```python
from build123d import *

# Parameters (mm, degrees)
SKETCH1_W                = 2
SKETCH1_H                = 27
M4_CLEARANCE_HOLE1_D     = 4.5
M4_CLEARANCE_HOLE1_DEPTH = 4.5
CUT_EXTRUDE1_START       = -10
CUT_EXTRUDE1_DEPTH       = 4
CIRPATTERN3_COUNT        = 6
SKETCH7_W                = 13.590111476
SKETCH7_H                = 85.87559673
CUT_EXTRUDE2_DEPTH       = 5
FILLET1_R                = 5
CUT_EXTRUDE3_DEPTH       = 46
BOSS_EXTRUDE1_START      = -9.8884
SKETCH8_3_R              = 2.45
BOSS_EXTRUDE1_DEPTH      = 1
BOSS_EXTRUDE2_START      = -8.8884
SKETCH8_4_R              = 2.45
BOSS_EXTRUDE2_DEPTH      = 4
BOSS_EXTRUDE3_DEPTH      = 37
BOSS_EXTRUDE4_START      = -2
SKETCH12_R               = 2.25
BOSS_EXTRUDE4_DEPTH      = 10


with BuildPart() as part:
    # Sketch1 → Revolve1 (revolve)
    with BuildSketch(Plane.XY):
        Polygon((32.5, 0), (39.5, 0), (52, 0), (52, 4.5), (39.5, 4.5), (39.5, 35), (42.5, 35), (42.5, 45), (32.5, 45), (32.5, 38), (32.5, 33), (32.5, 27), align=None)
        with Locations((31.5, 13.5)):
            Rectangle(SKETCH1_W, SKETCH1_H)
    revolve(axis=Axis((0, 0, 0), (0, 1, 0)))

    # M4 Clearance Hole1
    with Locations(Plane(origin=(0, 4.5, 0), x_dir=(1, 0, 0), z_dir=(0, 1, 0))):
        with Locations((45.75, 0)):
            m4_clearance_hole1 = Hole(M4_CLEARANCE_HOLE1_D / 2, depth=M4_CLEARANCE_HOLE1_DEPTH)

    # Sketch5 → M3 Clearance Hole1 (revolve, cut)
    with BuildSketch(Plane(origin=(35.7, 45, 0), x_dir=(0, 0, 1), z_dir=(1, 0, 0))):
        Polygon((0, 0), (0, 11.021463052), (1.7, 10), (1.7, 0), align=None)
    m3_clearance_hole1 = revolve(axis=Axis((35.7, 51.35, 0), (0, -1, 0)), mode=Mode.SUBTRACT)

    # Sketch4_2 → Cut-Extrude1 (cut)
    with BuildSketch(Plane(origin=(0, 45, 0), x_dir=(1, 0, 0), z_dir=(0, 1, 0)).offset(CUT_EXTRUDE1_START)):
        with BuildLine():
            Line((38.45, 1.58771324), (38.45, -1.58771324))
            Line((38.45, -1.58771324), (35.7, -3.175426481))
            Line((35.7, -3.175426481), (42.214154639, -4.920888955))
            ThreePointArc((42.214154639, -4.920888955), (42.428478479, -2.464592039), (42.5, 0))
            ThreePointArc((42.5, 0), (42.428478479, 2.464592039), (42.214154639, 4.920888955))
            Line((42.214154639, 4.920888955), (35.7, 3.175426481))
            Line((35.7, 3.175426481), (38.45, 1.58771324))
        make_face()
        Polygon((32.95, -1.58771324), (35.7, -3.175426481), (38.45, -1.58771324), (38.45, 1.58771324), (35.7, 3.175426481), (32.95, 1.58771324), align=None)
    cut_extrude1 = extrude(amount=-CUT_EXTRUDE1_DEPTH, mode=Mode.SUBTRACT)

    # CirPattern3: M4 Clearance Hole1, M3 Clearance Hole1, Cut-Extrude1 ×6 about axis
    cirpattern3_axis = Axis((0, 0, 0), (0, 1, 0))
    for i in range(1, CIRPATTERN3_COUNT):
        add(m4_clearance_hole1.rotate(cirpattern3_axis, i * 360 / CIRPATTERN3_COUNT), mode=Mode.SUBTRACT)
        add(m3_clearance_hole1.rotate(cirpattern3_axis, i * 360 / CIRPATTERN3_COUNT), mode=Mode.SUBTRACT)
        add(cut_extrude1.rotate(cirpattern3_axis, i * 360 / CIRPATTERN3_COUNT), mode=Mode.SUBTRACT)

    # Sketch7 → Cut-Extrude2 (cut)
    with BuildSketch(Plane.XZ):
        with Locations((0, -42.937798365)):
            Rectangle(SKETCH7_W, SKETCH7_H)
    extrude(amount=-CUT_EXTRUDE2_DEPTH, mode=Mode.SUBTRACT)

    # Fillet1
    fillet1_edges = [part.edges().sort_by_distance(p)[0] for p in [
        (-6.795055738, 2.5, -29.733436019),
        (-6.795055738, 2.25, -51.554119307),
        (6.795055738, 2.5, -29.733436019),
        (6.795055738, 2.25, -51.554119307),
    ]]
    fillet(fillet1_edges, radius=FILLET1_R)

    # Sketch8 → Cut-Extrude3 (cut, through all)
    with BuildSketch(Plane(origin=(0, 45, 0), x_dir=(1, 0, 0), z_dir=(0, 1, 0))):
        Polygon((-33.77753348, 6.841230885), (-24.786528121, 58.870086558), (-44.494427997, 62.275770406), (-53.485433356, 10.246914732), align=None)
    extrude(amount=-CUT_EXTRUDE3_DEPTH, mode=Mode.SUBTRACT)

    # Sketch8_3 → Boss-Extrude1 (add)
    with BuildSketch(Plane(origin=(0, 45, 0), x_dir=(1, 0, 0), z_dir=(0, 1, 0)).offset(BOSS_EXTRUDE1_START)):
        Polygon((-34.67678822, 54.490274326), (-25.808233276, 52.957716595), (-24.786528121, 58.870086558), (-33.655083065, 60.402644289), align=None)
        with Locations((-30.040674072, 57.240991616)):
            Circle(SKETCH8_3_R, mode=Mode.SUBTRACT)
        Polygon((-45.516133152, 56.363400443), (-36.647578207, 54.830842711), (-35.625873053, 60.743212674), (-44.494427997, 62.275770406), align=None)
        with Locations((-40.091703009, 58.977890378)):
            Circle(SKETCH8_3_R, mode=Mode.SUBTRACT)
        Polygon((-53.485433356, 10.246914732), (-44.616878412, 8.714357001), (-43.595173257, 14.626726964), (-52.463728201, 16.159284695), align=None)
        with Locations((-48.231287405, 11.876009674)):
            Circle(SKETCH8_3_R, mode=Mode.SUBTRACT)
        with BuildLine():
            Line((-41.699432083, 8.210198775), (-33.77753348, 6.841230885))
            Line((-33.77753348, 6.841230885), (-32.755828325, 12.753600847))
            Line((-32.755828325, 12.753600847), (-40.118843779, 14.025989228))
            ThreePointArc((-40.118843779, 14.025989228), (-41.01235693, 11.146146378), (-41.699432083, 8.210198775))
        make_face()
        with Locations((-38.180258468, 10.139110912)):
            Circle(SKETCH8_3_R, mode=Mode.SUBTRACT)
    extrude(amount=BOSS_EXTRUDE1_DEPTH)

    # Sketch8_4 → Boss-Extrude2 (add)
    with BuildSketch(Plane(origin=(0, 45, 0), x_dir=(1, 0, 0), z_dir=(0, 1, 0)).offset(BOSS_EXTRUDE2_START)):
        Polygon((-34.67678822, 54.490274326), (-25.808233276, 52.957716595), (-24.786528121, 58.870086558), (-33.655083065, 60.402644289), align=None)
        with Locations((-30.040674072, 57.240991616)):
            Circle(SKETCH8_4_R, mode=Mode.SUBTRACT)
        Polygon((-45.516133152, 56.363400443), (-36.647578207, 54.830842711), (-35.625873053, 60.743212674), (-44.494427997, 62.275770406), align=None)
        with Locations((-40.091703009, 58.977890378)):
            Circle(SKETCH8_4_R, mode=Mode.SUBTRACT)
        Polygon((-36.647578207, 54.830842711), (-34.67678822, 54.490274326), (-33.655083065, 60.402644289), (-35.625873053, 60.743212674), align=None)
        Polygon((-53.485433356, 10.246914732), (-44.616878412, 8.714357001), (-43.595173257, 14.626726964), (-52.463728201, 16.159284695), align=None)
        with Locations((-48.231287405, 11.876009674)):
            Circle(SKETCH8_4_R, mode=Mode.SUBTRACT)
        Polygon((-44.616878412, 8.714357001), (-42.646088424, 8.373788616), (-41.62438327, 14.286158579), (-43.595173257, 14.626726964), align=None)
        with BuildLine():
            Line((-41.699432083, 8.210198775), (-33.77753348, 6.841230885))
            Line((-33.77753348, 6.841230885), (-32.755828325, 12.753600847))
            Line((-32.755828325, 12.753600847), (-40.118843779, 14.025989228))
            ThreePointArc((-40.118843779, 14.025989228), (-41.01235693, 11.146146378), (-41.699432083, 8.210198775))
        make_face()
        with Locations((-38.180258468, 10.139110912)):
            Circle(SKETCH8_4_R, mode=Mode.SUBTRACT)
        with BuildLine():
            Line((-42.646088424, 8.373788616), (-41.699432083, 8.210198775))
            ThreePointArc((-41.699432083, 8.210198775), (-41.01235693, 11.146146378), (-40.118843779, 14.025989228))
            Line((-40.118843779, 14.025989228), (-41.62438327, 14.286158579))
            Line((-41.62438327, 14.286158579), (-42.646088424, 8.373788616))
        make_face()
    extrude(amount=BOSS_EXTRUDE2_DEPTH)

    # Sketch11 → Boss-Extrude3 (add)
    with BuildSketch(Plane.XZ):
        with BuildLine():
            Line((-27.313133013, -44.249212027), (-24.786528121, -58.870086558))
            Line((-24.786528121, -58.870086558), (-9.274181519, -49.813905189))
            ThreePointArc((-9.274181519, -49.813905189), (-11.110324868, -50.448789631), (-13.049848902, -50.335886241))
            ThreePointArc((-13.049848902, -50.335886241), (-20.409666288, -47.827246649), (-27.313133013, -44.249212027))
        make_face()
    extrude(amount=-BOSS_EXTRUDE3_DEPTH)

    # Sketch12 → Boss-Extrude4 (add)
    with BuildSketch(Plane(origin=(0, 37, 0), x_dir=(1, 0, 0), z_dir=(0, 1, 0)).offset(BOSS_EXTRUDE4_START)):
        with BuildLine():
            ThreePointArc((-6.795055738, 45.495897179), (-7.45890719, 47.985438456), (-9.274182045, 49.813905496))
            Line((-9.274182045, 49.813905496), (-24.786528121, 58.870086558))
            Line((-24.786528121, 58.870086558), (-30.655076171, 24.910164692))
            ThreePointArc((-30.655076171, 24.910164692), (-19.990871879, 34.067800655), (-6.795055738, 38.911145158))
            Line((-6.795055738, 38.911145158), (-6.795055738, 45.495897179))
        make_face()
        with Locations((-22.875, 39.620662223)):
            Circle(SKETCH12_R, mode=Mode.SUBTRACT)
    extrude(amount=BOSS_EXTRUDE4_DEPTH)


solid = part.part
```
Source: CAD feature listing. Evaluate the final solid. Frame: model axes, mm. A direction names the side the tool comes from. Round coordinates to 2 decimals unless told otherwise and drop trailing zeros. Loops run counter-clockwise (first coordinate to the right, second up) from the corner with the lowest first, then second, coordinate; pieces in that order, holes last.
1. Ray query, L1, parallel to Z at x = 0, y = 18; L2, parallel to Z at x = -16.5, y = 9.5; L3, parallel to Z at x = 14, y = 29. Return the intervals inside material, ascending.
2. Section query A-A on y = 12. Output: boundary loops of the cut face in (x, z).
3. Section query C-C on z = 9. Output: boundary loops of the cut face in (x, y), and give its area (3 significant figures).
4. Section query B-B on x = 45.75. Output: boundary loops of the cut face in (y, z).
5. Mould query, pull axis Z, two halves, no side actions, for faces 1 (the flat face through (21.93, 33.03, 30.66)), 2 (the flat face through (-37.794, 42.59, -7.535)), 3 (the cylindrical face through (26.33, 2.28, 44.84)), 4 (the flat face through (-19, 31, -32)). Classes: released by +Z, released by -Z, zero draft, split by the parting line, or undercut.
6. Section query D-D on x = 2. Output: boundary loops of the cut face in (y, z), and give its area (3 significant figures).
7. Access query for faces 5 (the flat face through (15.587, 33.028, -34.321)), 6 (the flat face through (-16.456, 33.028, 28.547)), 7 (the flat face through (-42, 36.112, -11)), 8 (the flat face through (-37.517, 33.028, 3.662)). Directions: +Z, -Z, +X, -X, +Y, -Y. A direction counts if a zero-diameter tool reaches every point of the face in a straight line with its end or side. Return the directions, or none.
8. Contact query for flat-ended pins moving along their axis: pin 1 (4 mm diameter, centred on x = -22.88, z = 39.62, fed in from +Y); pin 2 (3 mm diameter, centred on y = 31.5, z = 33.5, fed in from +X); pin 3 (1.5 mm diameter, centred on y = 5.5, z = 28, fed in from -X); pin 4 (2 mm diameter, centred on y = 22.5, z = 0, fed in from -X). Output: stop coordinate, or through.
Answers below:
1. L1: z = -39.5 to -30.5, 30.5 to 39.5
1. L2: z = -54.03 to -49.31, -35.89 to -25.65, 25.65 to 35.89
1. L3: z = -36.94 to -29.33, 29.33 to 36.94
2. outline: (-38.74, -7.7) - (-33.78, -6.84) - (-30.66, -24.91) arc R39.5 ccw (long way) to start; (-27.31, -44.25) - (-24.79, -58.87) - (-9.27, -49.81) arc R5 cw to (-13.05, -50.34) arc R52 cw to start; hole circle Ø61 at (0, 0)
3. outline: (-51.22, 0) - (-29.14, 0) - (-29.14, 27) - (-31.23, 27) - (-31.23, 45) - (-41.54, 45) - (-41.54, 35) - (-38.46, 35) - (-38.46, 4.5) - (-51.22, 4.5) - close; (29.14, 0) - (51.22, 0) - (51.22, 4.5) - (38.46, 4.5) - (38.46, 35) - (41.54, 35) - (41.54, 45) - (31.23, 45) - (31.23, 27) - (29.14, 27) - close
3. area: 940 mm2
4. outline: (0, -24.72) - (4.5, -24.72) - (4.5, -2.25) - (0, -2.25) - close; (0, 2.25) - (4.5, 2.25) - (4.5, 24.72) - (0, 24.72) - close
5. face 1: released by +Z
5. face 2: released by -Z
5. face 3: split by the parting line
5. face 4: undercut
6. outline: (0, 30.43) - (27, 30.43) - (27, 32.44) - (45, 32.44) - (45, 42.45) - (35, 42.45) - (35, 39.45) - (4.5, 39.45) - (4.5, 51.96) - (0, 51.96) - close; (5, -39.45) - (35, -39.45) - (35, -42.45) - (45, -42.45) - (45, -32.44) - (27, -32.44) - (27, -30.43) - (5, -30.43) - close
6. area: 811 mm2
7. face 5: +X
7. face 6: none
7. face 7: -Y
7. face 8: -X
8. pin 1: passes through
8. pin 2: stops at x = 23.04
8. pin 3: stops at x = -28.6
8. pin 4: stops at x = -39.5
